Check sheet for the drawn part. Datum: minimum x, y, z corner. Units: mm. A direction names the side the tool comes from. Give positions to 0.01 mm unless a question says otherwise; leave off trailing zeros. Loops run counter-clockwise (first coordinate to the right, second up) from the corner with the lowest first, then second, coordinate; pieces in that order, holes last. Notation, with made-up numbers: (6, 25) -> (23, 25) arc R22 cw to (23, 40) -> close; hole circle Ø6 at (67.25, -21.75). An arc over 180 degrees is marked (long way). One line per question, with ' | ' between items.
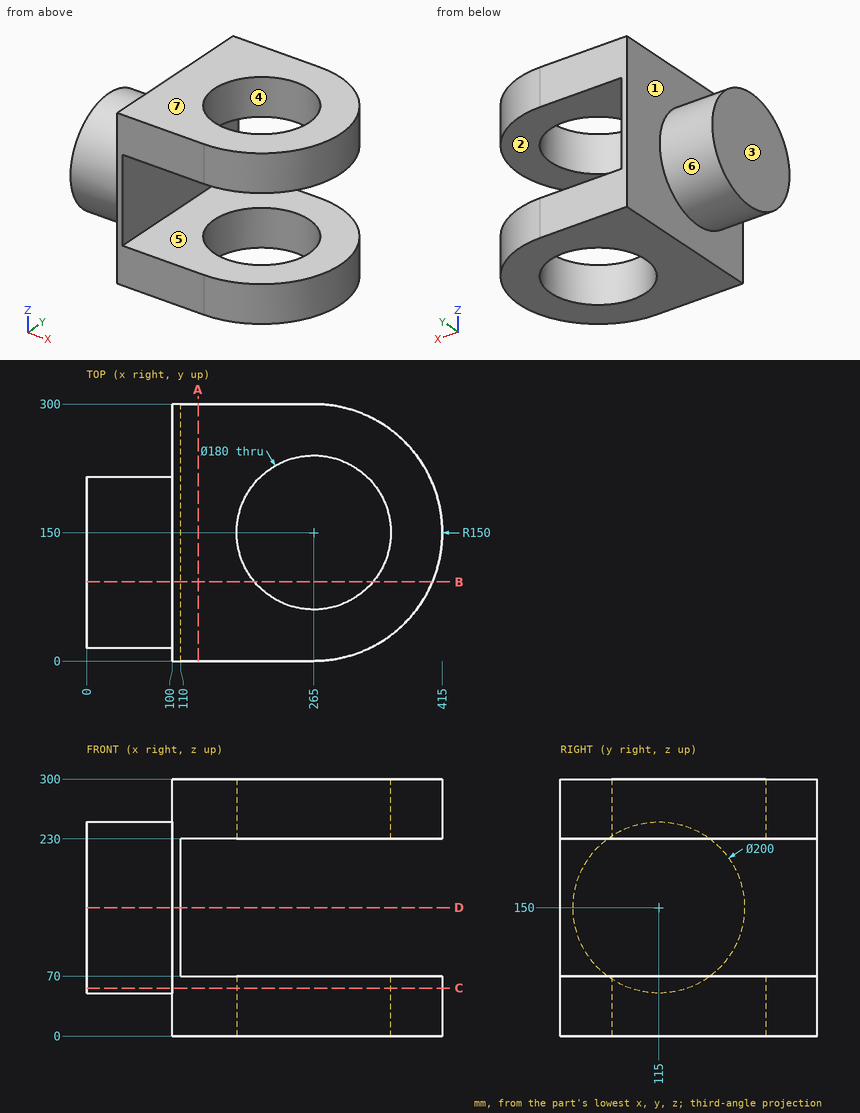
Item 1: Scan lines: probe 1 along X at (y, z) = (150, 281); probe 2 along Y at (x, z) = (265, 27); probe 3 along Z at (x, y) = (143, 196.5). Record each from-to range of solid material in increasing order.
Result:
probe 1: 100 to 175, 355 to 415 | probe 2: 0 to 60, 240 to 300 | probe 3: 0 to 70, 230 to 300
Item 2: Sectioned sample at C-C (z = 56). Record the cut outline in (x, y), plus the area to 3 significant figures.
Result:
outline: (0, 80.88) -> (100, 80.88) -> (100, 0) -> (265, 0) arc R150 ccw to (265, 300) -> (100, 300) -> (100, 149.12) -> (0, 149.12) -> close; hole circle Ø180 at (265, 150) | area: 66,200 mm2
Item 3: Depth check by flat-ended pin: pin 1 Ø2 at (y, z) = (257.5, 105.5) entering from -X; pin 2 Ø6 at (y, z) = (53, 241.5) entering from +X. Enter the tip coordinate at first touch or a pass-through.
Result:
pin 1: x = 100 | pin 2: x = 381.89
Item 4: Sectioned sample at B-B (y = 92.5). Record the cut outline in (x, z), plus the area to 3 significant figures.
Result:
outline: (0, 52.56) -> (100, 52.56) -> (100, 0) -> (195.76, 0) -> (195.76, 70) -> (110, 70) -> (110, 230) -> (195.76, 230) -> (195.76, 300) -> (100, 300) -> (100, 247.44) -> (0, 247.44) -> close; (334.24, 0) -> (403.54, 0) -> (403.54, 70) -> (334.24, 70) -> close; (334.24, 230) -> (403.54, 230) -> (403.54, 300) -> (334.24, 300) -> close | area: 44,200 mm2
Item 5: Sectioned sample at A-A (x = 130). Record the cut outline in (y, z).
Result:
outline: (0, 0) -> (300, 0) -> (300, 70) -> (0, 70) -> close; (0, 230) -> (300, 230) -> (300, 300) -> (0, 300) -> close
Item 6: Release check for a two-part mould opening along Z. For the marked faces 4, 5, 6 and 7 record: pulls with the +Z half, pulls with the -Z half, needs draft (parallel to the pull), parting line crosses it, or undercut.
Result:
face 4: needs draft | face 5: undercut | face 6: parting line crosses it | face 7: pulls with the +Z half
Item 7: Sectioned sample at D-D (z = 150). Record the cut outline in (x, y).
Result:
outline: (0, 15) -> (100, 15) -> (100, 0) -> (110, 0) -> (110, 300) -> (100, 300) -> (100, 215) -> (0, 215) -> close
Item 8: Set-up check for the marked faces 1, 2 and 3: record each of +Z, -Z, +X, -X, +Y, -Y from which the full face is reachable in a straight line by a thin tool's end or side.
Result:
face 1: -X | face 2: +X, +Y, -Y | face 3: +Z, -Z, -X, +Y, -Y
